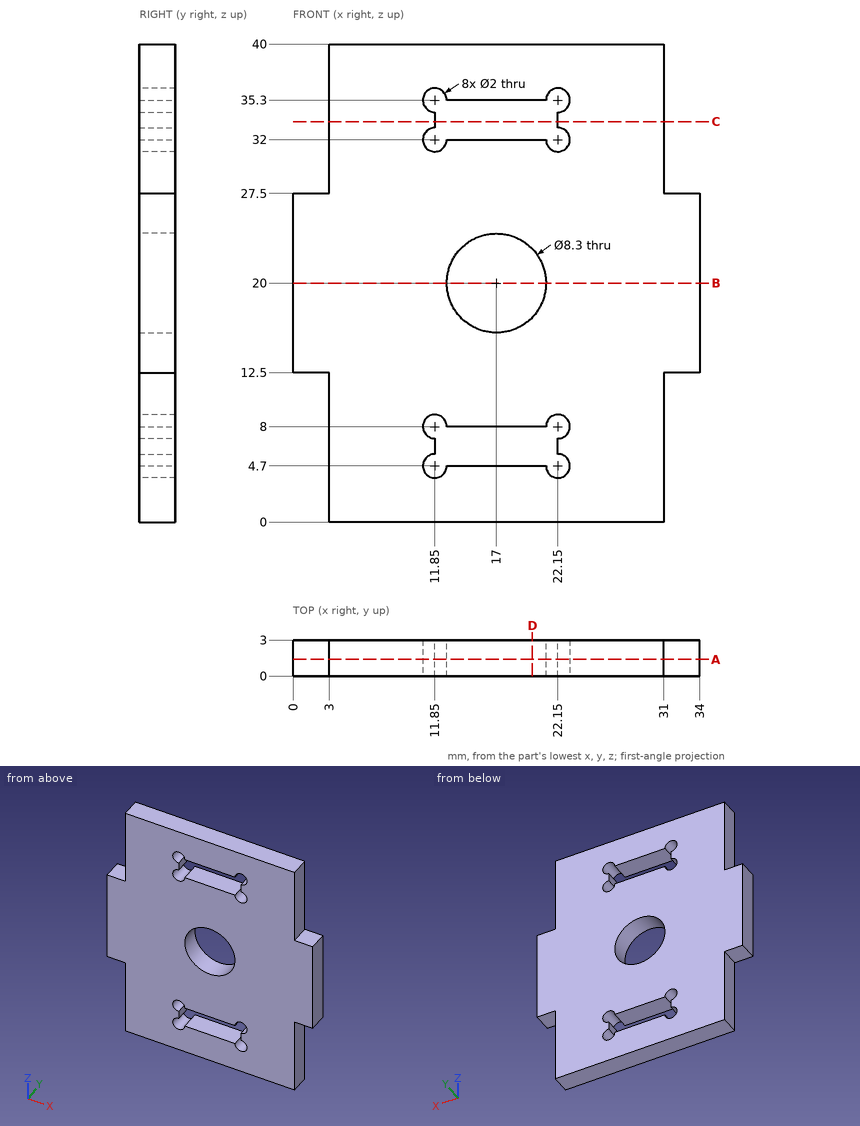
Part print with two shaded views. Sizes in mm from the minimum x, y, z corner. Give positions to 0.01 mm unless a question says otherwise; leave off trailing zeros. Order: outer loops, then holes, each group sorted by start corner. A loop starts at its lowest first (then second) coordinate and runs counter-clockwise, first axis right, second up.
1) Saw through at D-D, the plane x = 20. Write the cut outline in (y, z).
2) Saw through at C-C, the plane z = 33.5. Write the cut outline in (x, y).
3) Wall check: probe 1 along Z at (x, y) = (21.5, 0.25); probe 2 along Z at (x, y) = (14, 0.9); probe 3 along X at (y, z) = (1.65, 20). Give the ranges that are in metal, low to high.
4) Saw through at A-A, the plane y = 1.4. Count the separate pieces of the cut face and the enclosed holes in it, then the cut area to 3 significant figures.
5) Pin check, flat tips, straight feed: pin 1 (0.9 mm diameter, centred on x = 1.5, y = 1.5, fed in from -Z); pin 2 (1 mm diameter, centred on y = 1.5, z = 6, fed in from -X); pin 3 (0.9 mm diameter, centred on x = 32, y = 1.5, fed in from +Z). Stop position of each tip, or through.
6) Saw through at B-B, the plane z = 20. Write the cut outline in (x, y), then the cut area to 3 significant figures.
Computed:
1. outline: (0, 0) - (3, 0) - (3, 4.7) - (0, 4.7) - close; (0, 8) - (3, 8) - (3, 17.13) - (0, 17.13) - close; (0, 22.87) - (3, 22.87) - (3, 32) - (0, 32) - close; (0, 35.3) - (3, 35.3) - (3, 40) - (0, 40) - close
2. outline: (3, 0) - (11.85, 0) - (11.85, 3) - (3, 3) - close; (22.15, 0) - (31, 0) - (31, 3) - (22.15, 3) - close
3. probe 1: z = 0 to 3.94, 8.76 to 31.24, 36.06 to 40
3. probe 2: z = 0 to 4.7, 8 to 17.13, 22.87 to 32, 35.3 to 40
3. probe 3: x = 0 to 12.85, 21.15 to 34
4. separate pieces: 1
4. enclosed holes: 3
4. area: 1,070 mm2
5. pin 1: stops at z = 12.5
5. pin 2: stops at x = 3
5. pin 3: stops at z = 27.5
6. outline: (0, 0) - (12.85, 0) - (12.85, 3) - (0, 3) - close; (21.15, 0) - (34, 0) - (34, 3) - (21.15, 3) - close
6. area: 77.1 mm2
